Drawing for the job (mm, zero at the part's lowest x, y, z). A direction names the side the tool comes from. Give positions to 0.01 mm unless a question says otherwise; leave off trailing zeros. Order: outer loops, then holes, each group sorted by start corner. A loop starts at its lowest first (then second) coordinate and runs counter-clockwise, first axis right, second up. Notation, with made-up numbers: (30, 86) -> (36, 86) arc R20 cw to (36, 96) -> close; hole circle Ø10 at (53, 85). An arc over 180 degrees is marked (long way). Use a Markdown table: item, result. Add a question column.
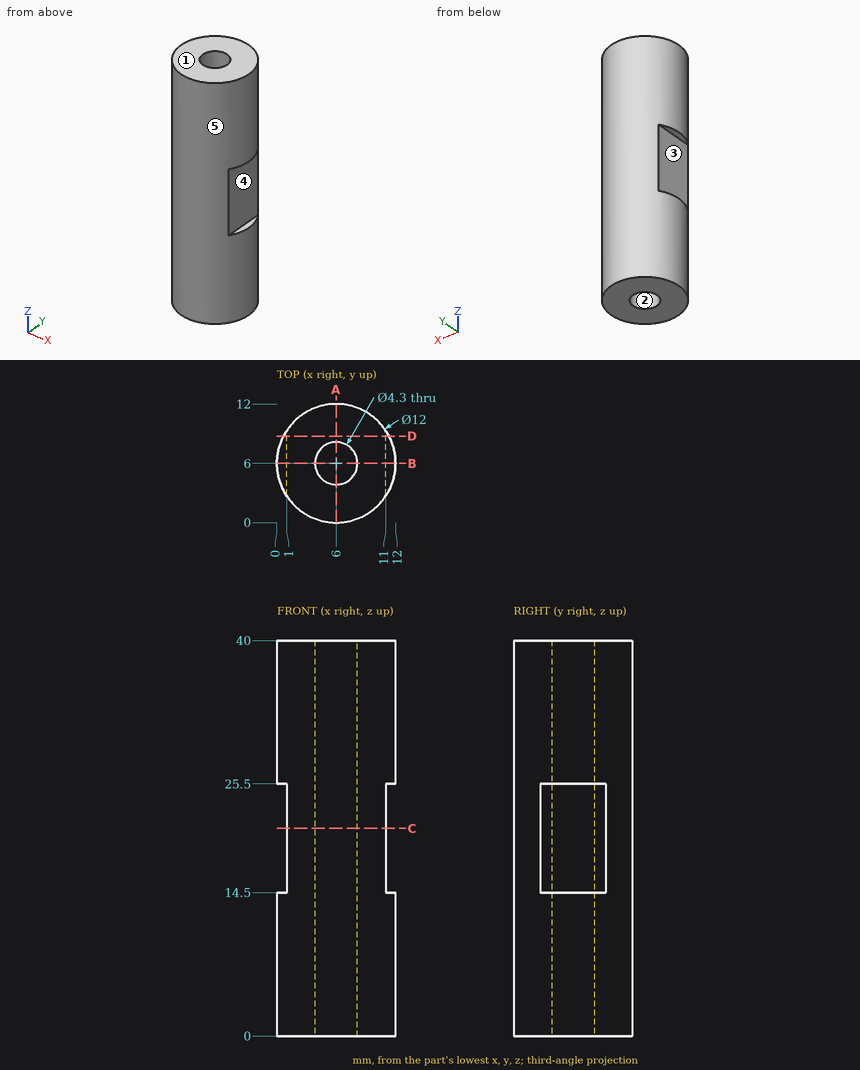
(1) Pin check, flat tips, straight feed: pin 1 Ø5 at (y, z) = (3, 9) entering from -X; pin 2 Ø5.5 at (y, z) = (6, 17.5) entering from +X; pin 3 Ø4 at (y, z) = (10, 29) entering from -X. Stop position of each tip, or through.
(2) Mould opens along Z. For the marked faces 1, 2 and 3 say: released by +Z, released by -Z, zero draft, split by the parting line, or undercut.
(3) Band-saw the part on A-A on x = 6. Give the cut face in (y, z), plus the area to 3 significant figures.
(4) Tool access for the marked faces 4 and 5: list every direction of +Z, -Z, +X, -X, +Y, -Y with a clear straight run to the whole face (end or side of a thin tool).
(5) Band-saw the part on D-D on y = 8.75. Give the cut face in (x, z), plus the area to 3 significant figures.
(6) Band-saw the part on C-C on z = 21. Give the cut face in (x, y).
(7) Band-saw the part on B-B on y = 6. Give the cut face in (x, z).
(8) Wall check: probe 1 along Y at (x, z) = (6, 14); probe 2 along Y at (x, z) = (6.75, 2); probe 3 along X at (y, z) = (8.5, 23). Give the ranges that are in metal, low to high.
Response:
| question | item | result |
|---|---|---|
| 1 | pin 1 | stops at x = 0.02 |
| 1 | pin 2 | stops at x = 11 |
| 1 | pin 3 | stops at x = 0.34 |
| 2 | face 1 | released by +Z |
| 2 | face 2 | zero draft |
| 2 | face 3 | undercut |
| 3 | outline | (0, 0) -> (3.85, 0) -> (3.85, 40) -> (0, 40) -> close; (8.15, 0) -> (12, 0) -> (12, 40) -> (8.15, 40) -> close |
| 3 | area | 308 mm² |
| 4 | face 4 | +X, +Y, -Y |
| 4 | face 5 | +Z, -Z |
| 5 | outline | (0.67, 0) -> (11.33, 0) -> (11.33, 14.5) -> (11, 14.5) -> (11, 25.5) -> (11.33, 25.5) -> (11.33, 40) -> (0.67, 40) -> (0.67, 25.5) -> (1, 25.5) -> (1, 14.5) -> (0.67, 14.5) -> close |
| 5 | area | 419 mm² |
| 6 | outline | (1, 2.68) arc R6 ccw to (11, 2.68) -> (11, 9.32) arc R6 ccw to (1, 9.32) -> close; hole circle Ø4.3 at (6, 6) |
| 7 | outline | (0, 0) -> (3.85, 0) -> (3.85, 40) -> (0, 40) -> (0, 25.5) -> (1, 25.5) -> (1, 14.5) -> (0, 14.5) -> close; (8.15, 0) -> (12, 0) -> (12, 14.5) -> (11, 14.5) -> (11, 25.5) -> (12, 25.5) -> (12, 40) -> (8.15, 40) -> close |
| 8 | probe 1 | y = 0 to 3.85, 8.15 to 12 |
| 8 | probe 2 | y = 0.05 to 3.99, 8.01 to 11.95 |
| 8 | probe 3 | x = 1 to 11 |
